Can you work these out from the drawing? Everything is in mm from the part's minimum corner. Round coordinates to 2 decimals unless told otherwise and drop trailing zeros. Loops run counter-clockwise (first coordinate to the right, second up) from the corner with the lowest first, then second, coordinate; pieces in that order, holes last. Notation, with made-up numbers: M 64.25,-16 L 89.25,-16 A10 cw 89.25,-1 Z; hole C -27,12.25 d7. An arc over 180 degrees is marked long. Answer in a Markdown table with one row per item.
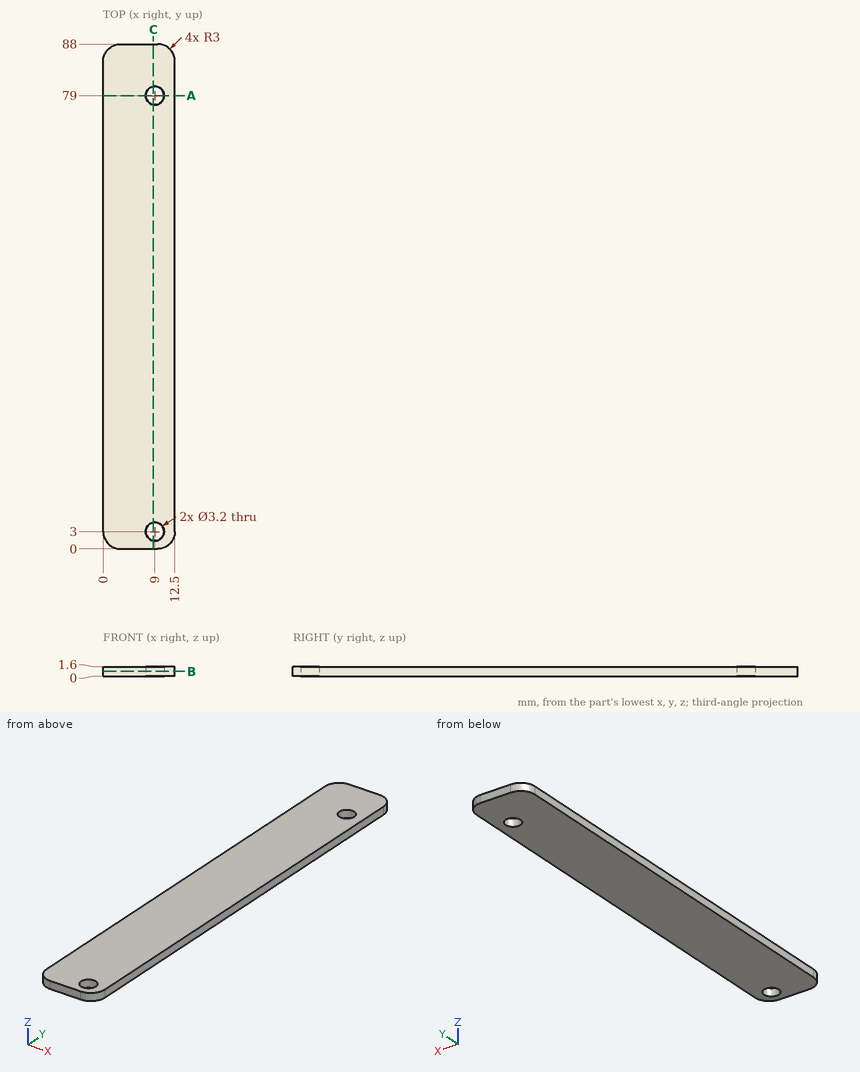
1) I want a section at B-B, the plane z = 0.8. Please give me the cut outline in (x, y), plus the area to 3 significant figures.
Computed:
| item | result |
|---|---|
| outline | M 0,3 A3 ccw 3,0 L 9.5,0 A3 ccw 12.5,3 L 12.5,85 A3 ccw 9.5,88 L 3,88 A3 ccw 0,85 Z; hole C 9,3 d3.2; hole C 9,79 d3.2 |
| area | 1,080 mm² |
2) I want a section at A-A, the plane y = 79. Please give me the cut outline in (x, z).
Computed:
| item | result |
|---|---|
| outline | M 0,0 L 7.4,0 L 7.4,1.6 L 0,1.6 Z; M 10.6,0 L 12.5,0 L 12.5,1.6 L 10.6,1.6 Z |
3) I want a section at C-C, the plane x = 8.75. Please give me the cut outline in (y, z), plus the area to 3 significant figures.
Computed:
| item | result |
|---|---|
| outline | M 0,0 L 1.42,0 L 1.42,1.6 L 0,1.6 Z; M 4.58,0 L 77.42,0 L 77.42,1.6 L 4.58,1.6 Z; M 80.58,0 L 88,0 L 88,1.6 L 80.58,1.6 Z |
| area | 131 mm² |
4) I need wall thicknesses on line 1 (Y direction, x = 9, z = 1.25); line 2 (X direction, y = 3, z = 0.95); line 3 (Y direction, x = 9.5, z = 0.15). Which ranges of each line are inside material? Lowest first, please.
Computed:
| item | result |
|---|---|
| line 1 | y = 0 to 1.4, 4.6 to 77.4, 80.6 to 88 |
| line 2 | x = 0 to 7.4, 10.6 to 12.5 |
| line 3 | y = 0 to 1.48, 4.52 to 77.48, 80.52 to 88 |
5) Will this pin go through, and if not, where does the flat tip stop? P1, Ø3.5, axis at x = 9, y = 3, coming from the +Z side.
Computed:
| item | result |
|---|---|
| P1 | stops at z = 1.6 |
